Verification items for the finished model (mm, model axes). A direction names the side the tool comes from. Round coordinates to 2 decimals unless told otherwise and drop trailing zeros. Write each loop counter-clockwise with the first axis right and the second up, starting at its lowest first coordinate (ties: lowest second). Pieces come first, ordered by that corner, then holes. Notation, with made-up numbers: (50, -11) -> (73, -11) arc R18 ccw to (73, -1) -> close; hole circle Ø5 at (61.25, 64). An arc over 180 degrees is marked (long way). Answer as a JSON object with one key per item and string values. Group by question number.
(1) Gauge pin test, flat ends, axial feed: pin 1 Ø0.7 at (y, z) = (1, 1) entering from -X; pin 2 Ø1 at (y, z) = (-2.5, 0.5) entering from -X; pin 3 Ø1 at (x, y) = (-1, -6) entering from +Z. Record the tip position at first contact, or that the pin passes through.
(2) Draft check along Z on faces 1 (the face through (1, 0, 1)), 2 (the face through (0.7, 1.1, -0.25)), 3 (the face through (-0.434, 0.412, 1.952)). Enter one of: released by +Z, released by -Z, zero draft, split by the parting line, or undercut.
(3) Sectioned sample at D-D on x = -1.4. Record the cut outline in (y, z).
(4) Sectioned sample at B-B on z = 0. Record the cut outline in (x, y).
(5) Sectioned sample at C-C on y = -4.75. Record the cut outline in (x, z).
(6) Sectioned sample at A-A on x = 0. Record the cut outline in (y, z).
(7) Set-up check for faces 4 (the face through (0.25, 1.1, -0.7)), 5 (the face through (0, -8, 0)), 6 (the face through (0, -4, 1)): record each of +Z, -Z, +X, -X, +Y, -Y from which the full face is reachable in a straight line by a thin tool's end or side.
(8) Scan lines: L1, parallel to Z at x = 0.75, y = 1.25; L2, parallel to Y at x = 1.7, z = 0.3; L3, parallel to X at y = 0.5, z = -1.3. Record each from-to range of solid material in increasing order. Write a range as from..to.
```python
from build123d import *

# Parameters (mm, degrees)
CUT_EXTRUDE1_START = -0.7
CUT_EXTRUDE1_DEPTH = 8.785281374


with BuildPart() as part:
    # Sketch1 → Revolve1 (revolve)
    with BuildSketch(Plane.XY, mode=Mode.PRIVATE) as revolve1_sk:
        with BuildLine():
            Line((-2, 0), (-1, 0))
            Line((-1, 0), (-1, -7.6))
            Line((-1, -7.6), (-0.6, -8))
            Line((-0.6, -8), (0, -8))
            Line((0, -8), (0, 1.6))
            ThreePointArc((0, 1.6), (-1.070466269, 1.402517077), (-2, 0.836067977))
            Line((-2, 0.836067977), (-2, 0))
        make_face()
    revolve(revolve1_sk.sketch.rotate(Axis((0, -8, 0), (0, 1, 0)), 180), axis=Axis((0, -8, 0), (0, 1, 0)))

    # Sketch2 → Cut-Extrude1 (cut, through all)
    with BuildSketch(Plane.XZ.offset(CUT_EXTRUDE1_START)):
        Polygon((-0.25, 1.15), (0.25, 1.15), (0.25, 0.25), (1.15, 0.25), (1.15, -0.25), (0.25, -0.25), (0.25, -1.15), (-0.25, -1.15), (-0.25, -0.25), (-1.15, -0.25), (-1.15, 0.25), (-0.25, 0.25), align=None)
    extrude(amount=-CUT_EXTRUDE1_DEPTH, mode=Mode.SUBTRACT)


solid = part.part
```
Computed values:
{
 "1": {"pin 1": "x = -1.88", "pin 2": "x = -1", "pin 3": "z = 0.87"},
 "2": {"face 1": "zero draft", "face 2": "undercut", "face 3": "split by the parting line"},
 "3": {"outline": "(0, -1.43) -> (0.84, -1.43) arc R2.65 ccw to (0.84, 1.43) -> (0, 1.43) -> close"},
 "4": {"outline": "(-2, 0) -> (-1, 0) -> (-1, -7.6) -> (-0.6, -8) -> (0.6, -8) -> (1, -7.6) -> (1, 0) -> (2, 0) -> (2, 0.84) arc R3 ccw to (1.15, 1.37) -> (1.15, 0.7) -> (-1.15, 0.7) -> (-1.15, 1.37) arc R3 ccw to (-2, 0.84) -> close"},
 "5": {"outline": "circle Ø2 at (0, 0)"},
 "6": {"outline": "(-8, -0.6) -> (-7.6, -1) -> (0, -1) -> (0, -2) -> (0.84, -2) arc R3 ccw to (1.37, -1.15) -> (0.7, -1.15) -> (0.7, 1.15) -> (1.37, 1.15) arc R3 ccw to (0.84, 2) -> (0, 2) -> (0, 1) -> (-7.6, 1) -> (-8, 0.6) -> close"},
 "7": {"face 4": "+Y", "face 5": "+Z, -Z, +X, -X, -Y", "face 6": "-Y"},
 "8": {"L1": "-1.19..-0.25, 0.25..1.19", "L2": "0..1.05", "L3": "-1.52..1.52"}
}
